Design review of the part built by this model. Coordinates are the model's own, in mm. Face numbers are marked on the shaded views. Round coordinates to 2 decimals unless told otherwise and drop trailing zeros. Write each loop counter-clockwise with the first axis right and the second up, starting at its lowest first coordinate (ties: lowest second). Pieces come first, ordered by that corner, then holes. Notation, with made-up numbers: M 35,0 L 53,0 A22 cw 53,36 Z; hole C 73,-11.5 d6. An arc over 180 degrees is marked long. Use CSV: the item, a comma, the result in double quotes.
from build123d import *

# Parameters (mm, degrees)
HOLE_WIZARD_M4_1_D     = 4
HOLE_WIZARD_M4_1_DEPTH = 6.1
HOLE_WIZARD_M4_1_TIP   = 1.201721238
HOLE_WIZARD_M3_1_D     = 3
HOLE_WIZARD_M3_1_DEPTH = 5.5
HOLE_WIZARD_M3_1_TIP   = 0.901290929
SKETCH_11_R            = 1
EXTRUDE_1_DEPTH        = 40
EXTRUDE_2_DEPTH        = 0.3
SKETCH_13_R            = 1
EXTRUDE_3_DEPTH        = 5
CUT_EXTRUDE_1_DEPTH    = 4
CUT_EXTRUDE_2_DEPTH    = 10


with BuildPart() as part:
    # 草图1 → 旋转1 (revolve)
    with BuildSketch(Plane(origin=(0, 0, 0), x_dir=(0, 0, -1), z_dir=(1, 0, 0)), mode=Mode.PRIVATE) as revolve_1_sk:
        Polygon((-2, 25), (-38, 25), (-43, 20), (-43, 3), (-65, 3), (-65, 0), (0, 0), (0, 3), (-2, 3), align=None)
    revolve(revolve_1_sk.sketch.rotate(Axis((0, 0, 0), (0, 0, 1)), 90), axis=Axis((0, 0, 0), (0, 0, 1)))

    # M4 螺纹孔1
    with Locations(Plane.XY.offset(43)):
        with Locations((0, 15), (15, 0), (0, -15), (-15, 0)):
            Hole(HOLE_WIZARD_M4_1_D / 2, depth=HOLE_WIZARD_M4_1_DEPTH)
            with Locations((0, 0, -(HOLE_WIZARD_M4_1_DEPTH + HOLE_WIZARD_M4_1_TIP / 2))):  # 118° drill point
                Cone(0, HOLE_WIZARD_M4_1_D / 2, HOLE_WIZARD_M4_1_TIP, mode=Mode.SUBTRACT)

    # M3 螺纹孔1
    with Locations(Plane(origin=(0, 0, 2), x_dir=(-1, 0, 0), z_dir=(0, 0, -1))):
        with Locations((0, 10), (10, 0), (0, -10), (-10, 0)):
            Hole(HOLE_WIZARD_M3_1_D / 2, depth=HOLE_WIZARD_M3_1_DEPTH)
            with Locations((0, 0, -(HOLE_WIZARD_M3_1_DEPTH + HOLE_WIZARD_M3_1_TIP / 2))):  # 118° drill point
                Cone(0, HOLE_WIZARD_M3_1_D / 2, HOLE_WIZARD_M3_1_TIP, mode=Mode.SUBTRACT)

    # 扫描1: sweep along a path in 草图9
    with BuildLine(Plane(origin=(0, 0, 0), x_dir=(0.7071067811865477, 0.7071067811865475, 0), z_dir=(-0.7071067811865475, 0.7071067811865477, 0))) as sweep_1_path:
        ThreePointArc((16, -43), (16.361695911, -44.147152873), (17.315959713, -44.879385242))
        ThreePointArc((17.315959713, -44.879385242), (19.138240785, -45.367663983), (21.017626027, -45.532088886))
    # 草图8 → 扫描1 (sweep)
    with BuildSketch(Plane.XY.offset(43)):
        Polygon((6.717514421, 13.788582233), (13.788582233, 6.717514421), (15.909902577, 8.838834765), (8.838834765, 15.909902577), align=None)
    sweep(path=sweep_1_path.line)

    # 草图11 → 凸台-拉伸1 (add)
    with BuildSketch(Plane(origin=(14.861705888, 14.861705888, 0), x_dir=(0, 0, -1), z_dir=(0.7071067811865476, 0.7071067811865476, 0))):
        with Locations(Location((-45.532088886, 0, 0), (0, 0, 270))):
            Circle(SKETCH_11_R)
        with Locations(Location((-45.532088886, 3, 0), (0, 0, 270))):
            Circle(SKETCH_11_R)
        with Locations(Location((-45.532088886, -3, 0), (0, 0, 270))):
            Circle(SKETCH_11_R)
    extrude(amount=EXTRUDE_1_DEPTH)

    # 草图12 → 凸台-拉伸2 (add)
    with BuildSketch(Plane(origin=(43.145977136, 43.145977136, 0), x_dir=(0, 0, -1), z_dir=(0.7071067811865477, 0.7071067811865475, 0))):
        Polygon((-47.032088886, -5), (-45.532088886, -5.866025404), (-44.032088886, -5), (-44.032088886, 5), (-45.532088886, 5.866025404), (-47.032088886, 5), align=None)
    extrude(amount=EXTRUDE_2_DEPTH)

    # 草图13 → 凸台-拉伸3 (add)
    # profile 1 of 3: a face of its own
    with BuildSketch(Plane(origin=(43.35810917, 43.35810917, 0), x_dir=(0, 0, -1), z_dir=(0.7071067811865477, 0.7071067811865475, -3.269036566852065e-15))):
        Polygon((-47.032088886, 5), (-47.032088886, -5), (-45.532088886, -5.866025404), (-44.032088886, -5), (-44.032088886, 5), (-45.532088886, 5.866025404), align=None)
        Polygon((-46.832088886, 4.884529946), (-46.832088886, -4.884529946), (-45.532088886, -5.635085296), (-44.232088886, -4.884529946), (-44.232088886, 4.884529946), (-45.532088886, 5.635085296), align=None, mode=Mode.SUBTRACT)
    # profile 2 of 3: a face of its own
    with BuildSketch(Plane(origin=(43.35810917, 43.35810917, 0), x_dir=(0, 0, -1), z_dir=(0.7071067811865477, 0.7071067811865475, -3.269036566852065e-15))):
        with Locations(Location((-45.532088886, 2, 0), (0, 0, 90))):
            Circle(SKETCH_13_R)
    # profile 3 of 3: a face of its own
    with BuildSketch(Plane(origin=(43.35810917, 43.35810917, 0), x_dir=(0, 0, -1), z_dir=(0.7071067811865477, 0.7071067811865475, -3.269036566852065e-15))):
        with Locations(Location((-45.532088886, -2, 0), (0, 0, 90))):
            Circle(SKETCH_13_R)
    extrude(amount=EXTRUDE_3_DEPTH)

    # 草图14 → 切除-拉伸1 (cut)
    with BuildSketch(Plane.XY.offset(61.8)):
        with BuildLine():
            Line((-2.45, 1.731328969), (-2.45, -1.731328969))
            ThreePointArc((-2.45, -1.731328969), (-3, 0), (-2.45, 1.731328969))
        make_face()
        with BuildLine():
            Line((2.45, 1.731328969), (2.45, -1.731328969))
            ThreePointArc((2.45, -1.731328969), (3, 0), (2.45, 1.731328969))
        make_face()
    extrude(amount=-CUT_EXTRUDE_1_DEPTH, mode=Mode.SUBTRACT)

    # 草图15 → 切除-拉伸2 (cut)
    with BuildSketch(Plane.XY.offset(53)):
        with BuildLine():
            Line((-2.45, -1.731328969), (-2.45, 1.731328969))
            ThreePointArc((-2.45, 1.731328969), (-3, 0), (-2.45, -1.731328969))
        make_face()
    extrude(amount=-CUT_EXTRUDE_2_DEPTH, mode=Mode.SUBTRACT)


solid = part.part
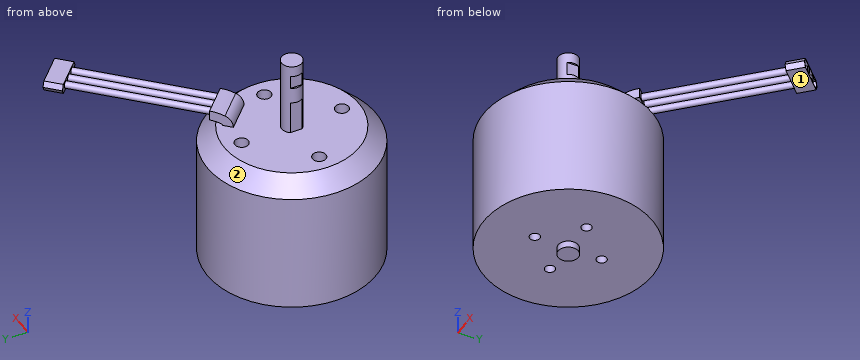
1) For pin 1 Ø8 at (y, z) = (25, 30.5) entering from -X; pin 2 Ø6 at (x, z) = (1.5, 49) entering from -Y; pin 3 Ø3.5 at (x, y) = (15, 0) entering from -Z, all flat-tipped, find the tip position at first contact; note any pin that passes through.
Answers:
pin 1,"x = -13.56"
pin 2,"y = -3"
pin 3,"z = 2"
2) The part is to be moulded in two halves that separate along Y. For the marked faces 1 and 2, say which applies: released by +Y, released by -Y, zero draft, split by the parting line, or undercut.
Answers:
face 1,"zero draft"
face 2,"split by the parting line"
3) Add section B-B on y = 28.5. Give the number of separate pieces and of enclosed holes in the cut face, then the cut area to 3 significant figures.
Answers:
separate pieces,"3"
enclosed holes,"0"
area,"13.3 mm²"
4) Add section A-A on z = 12. Write out the cut boundary in (x, y), then the cut area to 3 significant figures.
Answers:
outline,"C 0,0 d50"
area,"1,960 mm²"
5) Wall thickness on line 1 along Y through (x, z) = (0, 4.8); line 2 along X through (y, z) = (-15, 40); line 3 along Z through (x, y) = (6, -4): over which ranges is each line inside the solid? List them lowest first. Write a range as [from, to].
Answers:
line 1,"[-25, -11.5], [-8.5, 8.5], [11.5, 25]"
line 2,"[-17.44, -2], [2, 17.44]"
line 3,"[2, 43]"
